Can you work these out from the model? Positions are in its coordinate system, mm. Coordinates: 2 decimals unless noted, no trailing zeros. Write each loop counter-clockwise with the first axis right and the second up, starting at its lowest first coordinate (ties: lowest second). Pieces come first, ordered by that corner, then holes. Notation, with made-up numbers: (73, -17.5) -> (79, -17.5) arc R12 ccw to (79, 4.5) -> close; hole circle Ø10 at (-28.5, -39.5). An arc over 180 degrees is marked (long way). Use one line per item in the form item = value.
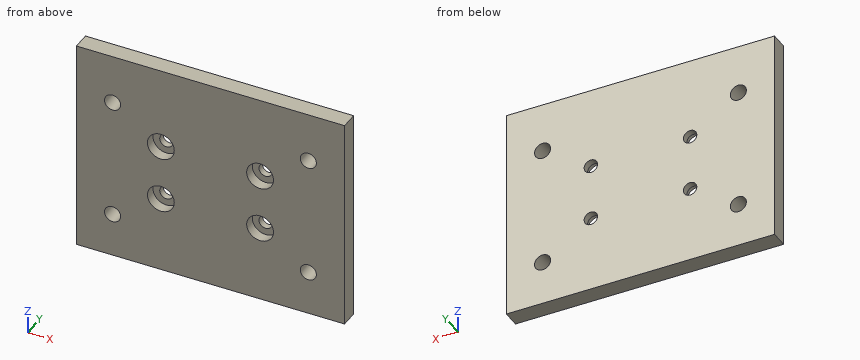
```python
from build123d import *

# Parameters (mm, degrees)
SKETCH001_W     = 100
SKETCH001_H     = 80
PAD_DEPTH       = 6.5
SKETCH004_R     = 2.5
POCKET_DEPTH    = 10
SKETCH_R        = 5
POCKET001_DEPTH = 4
SKETCH005_R     = 3
POCKET002_DEPTH = 10


with BuildPart() as part:
    # Sketch001 → Pad (new body)
    with BuildSketch(Plane.XZ):
        with Locations((0, 20.5)):
            Rectangle(SKETCH001_W, SKETCH001_H)
    extrude(amount=PAD_DEPTH)

    # Sketch004 → Pocket (cut)
    with BuildSketch(Plane(origin=(0, 0, 0), x_dir=(1, 0, 0), z_dir=(0, 1, 0))):
        with Locations((-18.5, -9)):
            Circle(SKETCH004_R)
        with Locations((18.5, -9)):
            Circle(SKETCH004_R)
        with Locations((-18.5, -30)):
            Circle(SKETCH004_R)
        with Locations((18.5, -30)):
            Circle(SKETCH004_R)
    extrude(amount=-POCKET_DEPTH, mode=Mode.SUBTRACT)

    # Sketch → Pocket001 (cut)
    with BuildSketch(Plane.XZ.offset(6.5)):
        with Locations((18.5, 9)):
            Circle(SKETCH_R)
        with Locations((18.5, 30)):
            Circle(SKETCH_R)
        with Locations((-18.5, 9)):
            Circle(SKETCH_R)
        with Locations((-18.5, 30)):
            Circle(SKETCH_R)
    extrude(amount=-POCKET001_DEPTH, mode=Mode.SUBTRACT)

    # Sketch005 → Pocket002 (cut)
    with BuildSketch(Plane.XZ.offset(6.5)):
        with Locations((36.5, -3)):
            Circle(SKETCH005_R)
        with Locations((36.5, 42)):
            Circle(SKETCH005_R)
        with Locations((-36.5, -3)):
            Circle(SKETCH005_R)
        with Locations((-36.5, 42)):
            Circle(SKETCH005_R)
    extrude(amount=-POCKET002_DEPTH, mode=Mode.SUBTRACT)


solid = part.part
```
Q1. Suppose I cut it at D-D (z = 30). Write out the boundary of the cut face in (x, y).
Return value:
outline = (-50, -6.5) -> (-23.5, -6.5) -> (-23.5, -2.5) -> (-21, -2.5) -> (-21, 0) -> (-50, 0) -> close; (-16, -2.5) -> (-13.5, -2.5) -> (-13.5, -6.5) -> (13.5, -6.5) -> (13.5, -2.5) -> (16, -2.5) -> (16, 0) -> (-16, 0) -> close; (21, -2.5) -> (23.5, -2.5) -> (23.5, -6.5) -> (50, -6.5) -> (50, 0) -> (21, 0) -> close
Q2. Suppose I cut it at B-B (x = 36.5). Write out the boundary of the cut face in (y, z), then the cut area to 3 significant figures.
Return value:
outline = (-6.5, -19.5) -> (0, -19.5) -> (0, -6) -> (-6.5, -6) -> close; (-6.5, 0) -> (0, 0) -> (0, 39) -> (-6.5, 39) -> close; (-6.5, 45) -> (0, 45) -> (0, 60.5) -> (-6.5, 60.5) -> close
area = 442 mm2
Q3. Will these pins go through, and if not, where does the flat tip stop? pin 1 (4 mm diameter, centred on x = 13, z = 52.5, fed in from +Y); pin 2 (8 mm diameter, centred on x = -18.5, z = 30, fed in from -Y).
Return value:
pin_1 = 0
pin_2 = -2.5
Q4. Suppose I cut it at A-A (z = 42). Write out the boundary of the cut face in (x, y).
Return value:
outline = (-50, -6.5) -> (-39.5, -6.5) -> (-39.5, 0) -> (-50, 0) -> close; (-33.5, -6.5) -> (33.5, -6.5) -> (33.5, 0) -> (-33.5, 0) -> close; (39.5, -6.5) -> (50, -6.5) -> (50, 0) -> (39.5, 0) -> close
Q5. Suppose I cut it at C-C (x = -18.5). Write out the boundary of the cut face in (y, z), then the cut area to 3 significant figures.
Return value:
outline = (-6.5, -19.5) -> (0, -19.5) -> (0, 6.5) -> (-2.5, 6.5) -> (-2.5, 4) -> (-6.5, 4) -> close; (-6.5, 14) -> (-2.5, 14) -> (-2.5, 11.5) -> (0, 11.5) -> (0, 27.5) -> (-2.5, 27.5) -> (-2.5, 25) -> (-6.5, 25) -> close; (-6.5, 35) -> (-2.5, 35) -> (-2.5, 32.5) -> (0, 32.5) -> (0, 60.5) -> (-6.5, 60.5) -> close
area = 415 mm2
Q6. If I drill on line 1 (X direction, y = -0.8, z = 9); line 2 (Z direction, x = -18.5, y = -0.7); line 3 (Z direction, x = -36.5, y = -2.75), over which ranges is the centre line in solid material (lowest first)? Write a range as from..to.
Return value:
line_1 = -50..-21, -16..16, 21..50
line_2 = -19.5..6.5, 11.5..27.5, 32.5..60.5
line_3 = -19.5..-6, 0..39, 45..60.5
